Verification items for this drawing (mm, ordinates from the low corner). A direction names the side the tool comes from. Coordinates: 2 decimals unless noted, no trailing zeros. Loops run counter-clockwise (first coordinate to the right, second up) from the corner with the lowest first, then second, coordinate; pieces in that order, holes last. Notation, with made-up numbers: M 79,80.5 L 104,80.5 A9 cw 104,97.5 Z; hole C 2,39.5 d10. An arc over 180 degrees is marked long. Write each question's results on one line, items separated by ' | '. Start each with the question number.
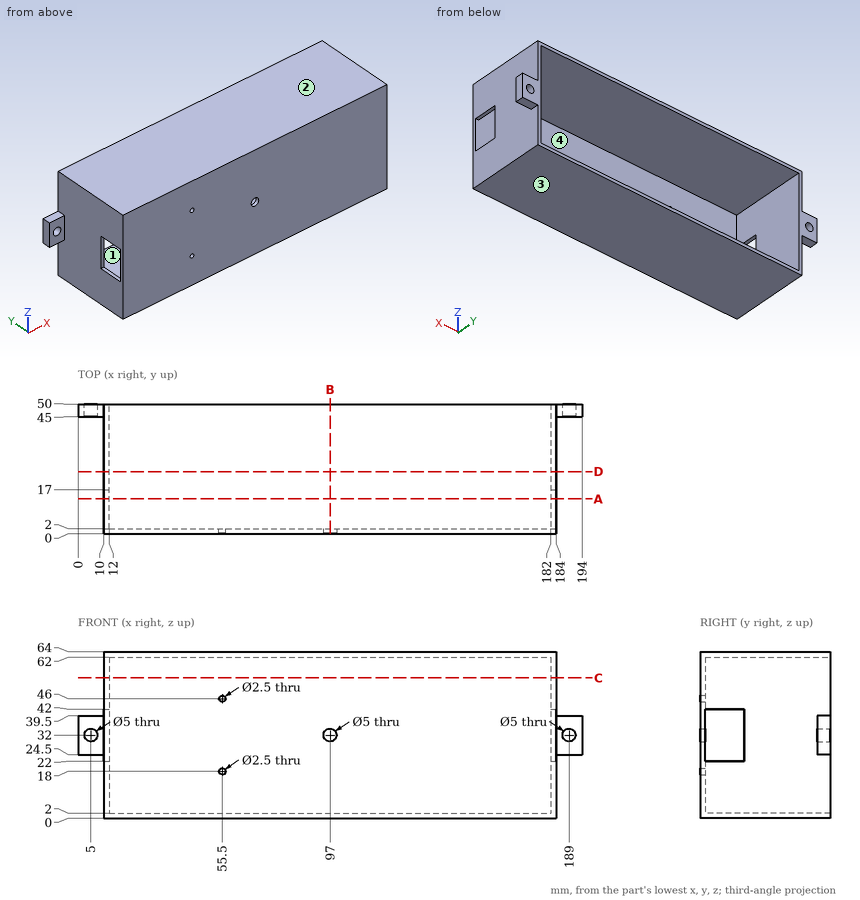
Item 1: Section check D-D (y = 24). Record the cut outline in (x, z).
Item 2: Thickness scan on line 1 (X direction, y = 46, z = 32); line 2 (X direction, y = 3, z = 3.5); line 3 (X direction, y = 0.9, z = 32). Record the ranges inside material, lowest first.
Item 3: Section check A-A (y = 13.5). Record the cut outline in (x, z), plus the area to 3 significant figures.
Item 4: Section check B-B (x = 97). Record the cut outline in (y, z).
Item 5: Section check C-C (z = 54). Record the cut outline in (x, y), plus the area to 3 significant figures.
Item 6: Release check for a two-part mould opening along X. For the marked faces 3 and 4 record: +X half, -X half, draft (parallel to the pull), parting line (faces both ways), or undercut.
Item 7: Tool access check on the marked faces 1 and 2. Record the directions out of +Z, -Z, +X, -X, +Y, -Y that give a thin tool (end or side, any length) a straight path to the whole face; none if there is none.
Item 8: Depth check by flat-ended pin: P1, Ø24, axis at y = 16.5, z = 38.5, coming from the -X side; P2, Ø12, axis at x = 116.5, z = 37.5, coming from the +Y side; P3, Ø6, axis at x = 5, z = 32, coming from the -Y side; P4, Ø4.5, axis at x = 97, z = 32, coming from the +Y side. Enter the tip coordinate at first touch or a pass-through.
Computed values:
1) outline: M 10,0 L 184,0 L 184,64 L 10,64 Z; hole M 12,2 L 182,2 L 182,62 L 12,62 Z
2) line 1: x = 0 to 2.5, 7.5 to 12, 182 to 186.5, 191.5 to 194 | line 2: x = 10 to 12, 182 to 184 | line 3: x = 10 to 94.5, 99.5 to 184
3) outline: M 10,0 L 184,0 L 184,22 L 182,22 L 182,2 L 12,2 L 12,22 L 10,22 Z; M 10,42 L 12,42 L 12,62 L 182,62 L 182,42 L 184,42 L 184,64 L 10,64 Z | area: 856 mm²
4) outline: M 0,0 L 50,0 L 50,2 L 2,2 L 2,29.5 L 0,29.5 Z; M 0,34.5 L 2,34.5 L 2,62 L 50,62 L 50,64 L 0,64 Z
5) outline: M 10,0 L 184,0 L 184,50 L 182,50 L 182,2 L 12,2 L 12,50 L 10,50 Z | area: 540 mm²
6) face 3: draft | face 4: undercut
7) face 1: +Y | face 2: +Z, +X, -X, +Y, -Y
8) P1: stops at x = 10 | P2: stops at y = 2 | P3: stops at y = 45 | P4: passes through
